Verification items for the finished model (mm, model axes). A direction names the side the tool comes from. Round coordinates to 2 decimals unless told otherwise and drop trailing zeros. Loops run counter-clockwise (first coordinate to the right, second up) from the corner with the lowest first, then second, coordinate; pieces in that order, holes last. Notation, with made-up numbers: (83, 10) -> (132, 10) arc R4 cw to (132, 17) -> close; hole circle Ø11 at (-22, -6). An arc over 180 degrees is marked (long way). Use a Markdown table: item, result. Add a question column.
```python
from build123d import *

# Parameters (mm, degrees)
SKETCH1_W               = 9
SKETCH1_H               = 9
BOSS_EXTRUDE1_DEPTH     = 108
SKETCH2_W               = 18
SKETCH2_H               = 8
BOSS_EXTRUDE2_DEPTH     = 4.5
SKETCH3_R               = 1.65
CUT_EXTRUDE1_DEPTH      = 1
CUT_EXTRUDE1_DEPTH_BACK = 10


with BuildPart() as part:
    # Sketch1 → Boss-Extrude1 (new body, symmetric)
    with BuildSketch(Plane.XY):
        Rectangle(SKETCH1_W, SKETCH1_H)
    extrude(amount=BOSS_EXTRUDE1_DEPTH, both=True)

    # Sketch2 → Boss-Extrude2 (add, symmetric)
    with BuildSketch(Plane(origin=(0, 0, 0), x_dir=(1, 0, 0), z_dir=(0, 1, 0))):
        with Locations((0, 83)):
            Rectangle(SKETCH2_W, SKETCH2_H)
        with Locations((0, -83)):
            Rectangle(SKETCH2_W, SKETCH2_H)
    extrude(amount=BOSS_EXTRUDE2_DEPTH, both=True)

    # Sketch3 → Cut-Extrude1 (cut, two sides)
    with BuildSketch(Plane(origin=(0, 4.5, 0), x_dir=(1, 0, 0), z_dir=(0, 1, 0))) as cut_extrude1_sk:
        with Locations((0, 6)):
            Circle(SKETCH3_R)
        with Locations((0, -6)):
            Circle(SKETCH3_R)
    extrude(amount=CUT_EXTRUDE1_DEPTH, mode=Mode.SUBTRACT)
    extrude(cut_extrude1_sk.sketch, amount=-CUT_EXTRUDE1_DEPTH_BACK, mode=Mode.SUBTRACT)


solid = part.part
```
1) Sectioned sample at C-C on z = -55.5. Enter the section's corners in (x, y), then the cut area to 3 significant figures.
2) Sectioned sample at A-A on x = -6.5. Enter the section's corners in (y, z), then the cut area to 3 significant figures.
3) Release check for a two-part mould opening along X. For faces 1 (the face through (-0.4, 0.1, 7.6)), 2 (the face through (-7, 0, 79)), 3 (the face through (4.5, 0, 98)), 4 (the face through (-4.5, 0, 1)) record: released by +X, released by -X, zero draft, split by the parting line, or undercut.
4) Go/stop test with flat-tipped pins: pin 1 (4.5 mm diameter, centred on y = 1.5, z = -102.5, fed in from -X); pin 2 (2 mm diameter, centred on x = -6.5, y = 1, fed in from +Z); pin 3 (2.5 mm diameter, centred on y = -2, z = -2, fed in from +X). Record where each tip stops, or that it passes through.
5) Access from +Z, -Z, +X, -X, +Y, -Y to the whole of each face (thin tool, end or side, straight path). Record for faces 5 (the face through (-7, 0, -87)), 6 (the face through (7, 0, 79)), 7 (the face through (4.5, 0, -97)), 8 (the face through (-4.5, 0, 98)).
6) Thickness scan on line 1 (Z direction, x = 0, y = 2.75); line 2 (X direction, y = -2.25, z = -6); line 3 (Z direction, x = 6, y = 1). Record the ranges inside material, lowest first.
7) Sectioned sample at B-B on y = -2.75. Enter the section's corners in (x, z), then the cut area to 3 significant figures.
Geometry results:
| question | item | result |
|---|---|---|
| 1 | outline | (-4.5, -4.5) -> (4.5, -4.5) -> (4.5, 4.5) -> (-4.5, 4.5) -> close |
| 1 | area | 81.0 mm^2 |
| 2 | outline | (-4.5, -87) -> (4.5, -87) -> (4.5, -79) -> (-4.5, -79) -> close; (-4.5, 79) -> (4.5, 79) -> (4.5, 87) -> (-4.5, 87) -> close |
| 2 | area | 144 mm^2 |
| 3 | face 1 | undercut |
| 3 | face 2 | zero draft |
| 3 | face 3 | released by +X |
| 3 | face 4 | released by -X |
| 4 | pin 1 | x = -4.5 |
| 4 | pin 2 | z = 87 |
| 4 | pin 3 | x = 4.5 |
| 5 | face 5 | -Z, -X, +Y, -Y |
| 5 | face 6 | +X, +Y, -Y |
| 5 | face 7 | -Z, +X, +Y, -Y |
| 5 | face 8 | +Z, -X, +Y, -Y |
| 6 | line 1 | -108 to -7.65, -4.35 to 4.35, 7.65 to 108 |
| 6 | line 2 | -4.5 to -1.65, 1.65 to 4.5 |
| 6 | line 3 | -87 to -79, 79 to 87 |
| 7 | outline | (-9, -87) -> (-4.5, -87) -> (-4.5, -108) -> (4.5, -108) -> (4.5, -87) -> (9, -87) -> (9, -79) -> (4.5, -79) -> (4.5, 79) -> (9, 79) -> (9, 87) -> (4.5, 87) -> (4.5, 108) -> (-4.5, 108) -> (-4.5, 87) -> (-9, 87) -> (-9, 79) -> (-4.5, 79) -> (-4.5, -79) -> (-9, -79) -> close; hole circle Ø3.3 at (0, -6); hole circle Ø3.3 at (0, 6) |
| 7 | area | 2,070 mm^2 |
